The listing builds one solid part. Answer for the finished solid, in the listing's coordinates (mm). Face numbers are marked on the shaded views. Coordinates: 2 decimals unless noted, no trailing zeros. Write each loop counter-clockwise with the first axis right and the second up, starting at its lowest first coordinate (ties: lowest second). Pieces come first, ordered by that corner, then holes. Notation, with made-up numbers: M -11.5,-8.75 L 6.5,-8.75 A11 ccw 6.5,-3.75 Z; hole C -7,30.25 d3. An arc over 180 degrees is marked long. Answer as CSV lines item,"result".
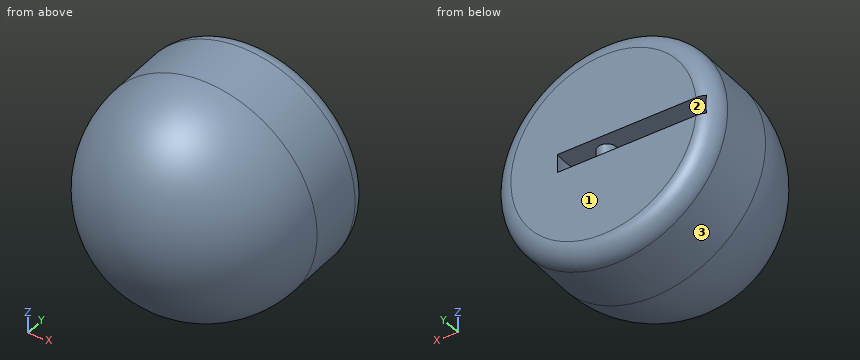
```python
from build123d import *

# Parameters (mm, degrees)
CUT_EXTRUDE_2_DEPTH = 1
SKETCH_3_R          = 1
EXTRUDE_2_DEPTH     = 2


with BuildPart() as part:
    # 草图1 → 旋转1 (revolve)
    with BuildSketch(Plane.XY, mode=Mode.PRIVATE) as revolve_1_sk:
        with BuildLine():
            Line((0, 6.040955631), (10, 6.040955631))
            ThreePointArc((10, 6.040955631), (11.414213562, 5.455169194), (12, 4.040955631))
            Line((12, 4.040955631), (12, -1.959044369))
            ThreePointArc((12, -1.959044369), (8.485281374, -10.444325743), (0, -13.959044369))
            Line((0, -13.959044369), (0, 6.040955631))
        make_face()
    revolve(revolve_1_sk.sketch.rotate(Axis((0, -13.959044369, 0), (0, 1, 0)), 90), axis=Axis((0, -13.959044369, 0), (0, 1, 0)))

    # 草图2 → 切除-拉伸2 (cut, symmetric)
    with BuildSketch(Plane.XY):
        with BuildLine():
            Line((5, 6.040955631), (-10, 6.040955631))
            ThreePointArc((-10, 6.040955631), (-10.461704233, 5.986933329), (-10.89846614, 5.827784833))
            ThreePointArc((-10.89846614, 5.827784833), (-2.829997478, -2.95832534), (5, 6.040955631))
        make_face()
    extrude(amount=CUT_EXTRUDE_2_DEPTH, both=True, mode=Mode.SUBTRACT)

    # 草图3 → 凸台-拉伸2 (add)
    with BuildSketch(Plane.XY.offset(-1)):
        with Locations(Location((-3, 1.040955631, 0), (0, 0, 180))):
            Circle(SKETCH_3_R)
        with Locations(Location((1, 4.040955631, 0), (0, 0, 180))):
            Circle(SKETCH_3_R)
    extrude(amount=EXTRUDE_2_DEPTH)


solid = part.part
```
Q1. Find section D-D (y = -6.5). Give the vertices of the cut face in (x, z), and give its area (3 significant figures).
Output:
outline,"C 0,0 d22.22"
area,"388 mm2"
Q2. Flat-ended cylindrical pins translate along their axes: pin 1 Ø5 at (x, z) = (-0.5, 4.5) entering from -Y; pin 2 Ø10 at (y, z) = (-1.5, -6) entering from +X; pin 3 Ø6 at (x, z) = (-4.5, 0.5) entering from -Y. Find the tip coordinate at first contact, or state that the pin passes through.
Output:
pin 1,"y = -13.79"
pin 2,"x = 11.96"
pin 3,"y = -13.86"
Q3. The mould has two halves that part along Y. Classify the marked faces 1, 2 and 3: pulls with the +Y half, pulls with the -Y half, needs draft (parallel to the pull), parting line crosses it, or undercut.
Output:
face 1,"pulls with the +Y half"
face 2,"undercut"
face 3,"needs draft"
Q4. Straight lines are drawn through the part: line 1 (X direction, y = 3.75, z = -0.75); line 2 (Z direction, x = -8.5, y = 3.5); line 3 (Y direction, x = -5.5, z = -5). For each, find the intervals that lie inside material, in ascending order.
Output:
line 1,"-11.98 to -10.83, 0.04 to 1.96, 4.96 to 11.98"
line 2,"-8.47 to -1, 1 to 8.47"
line 3,"-11.38 to 6.04"
Q5. Find section A-A (z = 0). Give the vertices of the cut face in (x, y).
Output:
outline,"M -12,-1.96 A12 ccw 12,-1.96 L 12,4.04 A2 ccw 10,6.04 L 5,6.04 A8 cw long -10.9,5.83 A2 ccw -12,4.04 Z; C -3,1.04 d2; C 1,4.04 d2"
Q6. Find section C-C (y = -11.25). Give the vertices of the cut face in (x, z).
Output:
outline,"C 0,0 d15.19"
Q7. Find section B-B (y = -2.5). Give the vertices of the cut face in (x, z).
Output:
outline,"C 0,0 d23.98; hole M -5.61,-1 L -0.27,-1 L -0.27,1 L -5.61,1 Z"
